Can you work these out from the model? Positions are in its coordinate system, mm. A direction names the side the tool comes from. Coordinates: 2 decimals unless noted, no trailing zeros. Order: outer loops, then holes, each group sorted by start corner. A loop starts at its lowest first (then second) coordinate and runs counter-clockwise, first axis right, second up. Notation, with made-up numbers: (83, 32.25) - (127, 32.25) arc R25 cw to (127, 46.25) - close; hole circle Ø4 at (-33, 50). An arc over 180 degrees is marked (long way). Use a Markdown table: item, result. Add a question column.
(1) I want a section at B-B (z = 0.25). List the corners of the cut face in (x, y) for me (3 decimals).
(2) For pin 1 Ø4 at (x, y) = (0.5, 4) entering from +Z (3 decimals); pin 2 Ø4 at (x, z) = (4.5, -4.5) entering from -Y; pin 3 Ø3 at (x, y) = (-6, 14) entering from +Z; pin 4 Ø8 at (x, z) = (3.5, 0.5) entering from -Y, each with a flat end and sliding along its axis, tell me the tip position at first contact or that it passes through.
(3) If I drill on L1, parallel to Y at x = 3.5, z = 2.25; L2, parallel to X at y = 15.25, z = 0; L3, parallel to X at y = 4, z = 0 (3 decimals), over which ranges is the centre line in solid material (lowest first)? Write a range as [from, to].
(4) We'd pull the mould along Z, two halves only. Please class faces 1 (the cylindrical face through (2.8, 3.1, -1.5)), 2 (the flat face through (-3, 6.35, 2)), 3 (the flat face through (-2.05, 20.02, -1.21)): pulls with the +Z half, pulls with the -Z half, needs draft (parallel to the pull), parting line crosses it, or undercut.
(5) I want a section at D-D (z = 4). List the corners of the cut face in (x, y) for me, and give its area (3 significant figures).
(6) On a 3-axis mill with a long thin cutter (end or side, diameter ignored), from which of +Z, -Z, +X, -X, +Y, -Y can I reach the whole of each face in a straight line? I mean faces 4 (the flat face through (-7, 19.05, 0)), 5 (the flat face through (-2, 21.59, 2)), 6 (the flat face through (0, 20, 2.381)). Say none if no direction works.
(7) I want a section at C-C (y = 17.25). List the corners of the cut face in (x, z) for me.
```python
from build123d import *

# Parameters (mm, degrees)
CUT_EXTRUDE1_DEPTH = 3.175


with BuildPart() as part:
    # Sketch1 → Revolve1 (revolve)
    with BuildSketch(Plane(origin=(0, 0, 0), x_dir=(0, 0, -1), z_dir=(1, 0, 0)), mode=Mode.PRIVATE) as revolve1_sk:
        Polygon((0, 0), (0, 21.59), (-7.9375, 21.59), (-7.9375, 19.05), (-6.35, 19.05), (-6.35, 6.35), (-3.175, 6.35), (-3.175, 0), align=None)
    revolve(revolve1_sk.sketch.rotate(Axis((0, 0, 0), (0, 1, 0)), 180), axis=Axis((0, 0, 0), (0, 1, 0)))

    # Sketch2 → Cut-Extrude1 (cut)
    with BuildSketch(Plane(origin=(0, 21.59, 0), x_dir=(1, 0, 0), z_dir=(0, 1, 0))):
        Polygon((-1.374815329, 2.38125), (-2.749630657, 0), (-1.374815329, -2.38125), (1.374815329, -2.38125), (2.749630657, 0), (1.374815329, 2.38125), align=None)
    extrude(amount=-CUT_EXTRUDE1_DEPTH, mode=Mode.SUBTRACT)


solid = part.part
```
Answers follow:
| question | item | result |
|---|---|---|
| 1 | outline | (-7.934, 19.05) - (-6.345, 19.05) - (-6.345, 6.35) - (-3.165, 6.35) - (-3.165, 0) - (3.165, 0) - (3.165, 6.35) - (6.345, 6.35) - (6.345, 19.05) - (7.934, 19.05) - (7.934, 21.59) - (2.605, 21.59) - (2.605, 18.415) - (-2.605, 18.415) - (-2.605, 21.59) - (-7.934, 21.59) - close |
| 2 | pin 1 | stops at z = 3.175 |
| 2 | pin 2 | stops at y = 6.35 |
| 2 | pin 3 | stops at z = 4.48 |
| 2 | pin 4 | stops at y = 0 |
| 3 | L1 | y = [6.35, 21.59] |
| 3 | L2 | x = [-6.35, 6.35] |
| 3 | L3 | x = [-3.175, 3.175] |
| 4 | face 1 | parting line crosses it |
| 4 | face 2 | needs draft |
| 4 | face 3 | undercut |
| 5 | outline | (-6.86, 19.05) - (-4.93, 19.05) - (-4.93, 6.35) - (4.93, 6.35) - (4.93, 19.05) - (6.86, 19.05) - (6.86, 21.59) - (-6.86, 21.59) - close |
| 5 | area | 160 mm² |
| 6 | face 4 | -Y |
| 6 | face 5 | +Z, -Z, +X, -X, +Y |
| 6 | face 6 | +Y |
| 7 | outline | circle Ø12.7 at (0, 0) |
